Here's how the part is built. I have some questions about the finished solid (model axes, mm). Coordinates: 2 decimals unless noted, no trailing zeros. Loops run counter-clockwise (first coordinate to the right, second up) from the corner with the lowest first, then second, coordinate; pieces in that order, holes last. Notation, with made-up numbers: (75.25, -24.75) -> (115.25, -24.75) arc R31 ccw to (115.25, 0.25) -> close; hole circle Ø3 at (58.25, 20). An arc over 180 degrees is marked (long way). Answer as a JSON object with one key per item and string values. Group by question number.
Q1. I want a section at B-B on y = 38.8. Write out the boundary of the cut face in (x, z), then the cut area to 3 significant figures.
Q2. I need wall thicknesses on line 1 (X direction, y = 38.8, z = 46.5); line 2 (Y direction, x = 69.5, z = 51.25) (3 decimals); line 3 (Y direction, x = 61.5, z = 47.5) (3 decimals). Which ranges of each line are inside material? Lowest first, please.
Q3. Thinking about a two-plate mould opening in X: for faces 1 (the flat face through (-21.6, 27.77, 49.89)), 2 (the flat face through (1.96, 27.77, 49.89)), 3 (the flat face through (-3, 43.5, 50)), 4 (the flat face through (56.94, 27.77, 49.89)), which applies, released by +X, released by -X, zero draft, split by the parting line, or undercut?
Q4. I want a section at A-A on x = 60.5. Write out the boundary of the cut face in (y, z) (3 decimals).
Q5. I'm going to push flat-ended pins straight in: pin 1 (0.9 mm diameter, centred on x = 27.5, z = 49, fed in from -Y) (3 decimals); pin 2 (1 mm diameter, centred on y = 28.5, z = 51, fed in from -X). Where does each tip first touch, or does it pass through?
Q6. I want a section at C-C on z = 47.5. Count the separate pieces of the cut face and the enclosed holes in it, then the cut area to 3 significant figures.
```python
from build123d import *

# Parameters (mm, degrees)
F_17_START                                     = 42.4
F_17_RACK_TEETH_MODULE_2_5_AND_20_DEGREE_DEPTH = 15.2
TWO_START                                      = 42.4
SKETCH2_R                                      = 2.15
TWO_CROSSHEAD_JOINT_THROUGH_HOLES_DEPTH        = 15.2


with BuildPart() as part:
    # Sketch1 → 17 rack teeth - module 2.5 and 20 degrees (new body)
    with BuildSketch(Plane.XY.offset(F_17_START)):
        Polygon((-80, 43.5), (-80, 30.625), (-73.686737096, 30.625), (-71.639404529, 25), (-69.732264883, 25), (-67.684932315, 30.625), (-65.832755462, 30.625), (-63.785422895, 25), (-61.878283249, 25), (-59.830950681, 30.625), (-57.978773828, 30.625), (-55.931441261, 25), (-54.024301615, 25), (-51.976969047, 30.625), (-50.124792194, 30.625), (-48.077459627, 25), (-46.170319981, 25), (-44.122987413, 30.625), (-42.27081056, 30.625), (-40.223477993, 25), (-38.316338347, 25), (-36.269005779, 30.625), (-34.416828926, 30.625), (-32.369496359, 25), (-30.462356713, 25), (-28.415024145, 30.625), (-26.562847292, 30.625), (-24.515514725, 25), (-22.608375079, 25), (-20.561042511, 30.625), (-18.708865659, 30.625), (-16.661533091, 25), (-14.754393445, 25), (-12.707060877, 30.625), (-10.854884025, 30.625), (-8.807551457, 25), (-6.900411811, 25), (-4.853079243, 30.625), (-3.000902391, 30.625), (-0.953569823, 25), (0.953569823, 25), (3.000902391, 30.625), (4.853079243, 30.625), (6.900411811, 25), (8.807551457, 25), (10.854884025, 30.625), (12.707060877, 30.625), (14.754393445, 25), (16.661533091, 25), (18.708865659, 30.625), (20.561042511, 30.625), (22.608375079, 25), (24.515514725, 25), (26.562847292, 30.625), (28.415024145, 30.625), (30.462356713, 25), (32.369496359, 25), (34.416828926, 30.625), (36.269005779, 30.625), (38.316338347, 25), (40.223477993, 25), (42.27081056, 30.625), (44.122987413, 30.625), (46.170319981, 25), (48.077459627, 25), (50.124792194, 30.625), (51.976969047, 30.625), (54.024301615, 25), (55.931441261, 25), (57.978773828, 30.625), (72, 30.625), (72, 43.5), align=None)
    extrude(amount=F_17_RACK_TEETH_MODULE_2_5_AND_20_DEGREE_DEPTH)

    # Sketch2 → Two crosshead joint through holes (cut)
    with BuildSketch(Plane.XY.offset(TWO_START)):
        with Locations(Location((60.5, 38.8, 0), (0, 0, 180))):
            Circle(SKETCH2_R)
        with Locations(Location((69.5, 38.8, 0), (0, 0, 180))):
            Circle(SKETCH2_R)
    extrude(amount=TWO_CROSSHEAD_JOINT_THROUGH_HOLES_DEPTH, mode=Mode.SUBTRACT)


solid = part.part
```
Result set:
{
 "1": {"outline": "(-80, 42.4) -> (58.35, 42.4) -> (58.35, 57.6) -> (-80, 57.6) -> close; (62.65, 42.4) -> (67.35, 42.4) -> (67.35, 57.6) -> (62.65, 57.6) -> close; (71.65, 42.4) -> (72, 42.4) -> (72, 57.6) -> (71.65, 57.6) -> close", "area": "2,180 mm²"},
 "2": {"line 1": "x = -80 to 58.35, 62.65 to 67.35, 71.65 to 72", "line 2": "y = 30.625 to 36.65, 40.95 to 43.5", "line 3": "y = 30.625 to 36.897, 40.703 to 43.5"},
 "3": {"face 1": "undercut", "face 2": "undercut", "face 3": "zero draft", "face 4": "released by +X"},
 "4": {"outline": "(30.625, 42.4) -> (36.65, 42.4) -> (36.65, 57.6) -> (30.625, 57.6) -> close; (40.95, 42.4) -> (43.5, 42.4) -> (43.5, 57.6) -> (40.95, 57.6) -> close"},
 "5": {"pin 1": "stops at y = 30.625", "pin 2": "stops at x = -73.1"},
 "6": {"separate pieces": "1", "enclosed holes": "2", "area": "2,310 mm²"}
}
